```python
from build123d import *

# Parameters (mm, degrees)
CUT_EXTRUDE1_DEPTH = 2.413


with BuildPart() as part:
    # Sketch3 → Revolve1 (revolve)
    with BuildSketch(Plane(origin=(0, 0, 0), x_dir=(0, 0, -1), z_dir=(1, 0, 0))):
        Polygon((10.3505, 0), (-10.3505, 0), (-10.3505, 3.48615), (-9.8679, 3.96875), (-6.0071, 3.96875), (-5.5245, 3.48615), (-5.5245, 2.413), (9.609666667, 2.413), (10.3505, 1.672166667), align=None)
    revolve(axis=Axis((0, 0, -10.3505), (0, 0, 1)))

    # Sketch4 → Cut-Extrude1 (cut)
    with BuildSketch(Plane.XY.offset(10.3505)):
        Polygon((0, -2.291358881), (1.984375, -1.14567944), (1.984375, 1.14567944), (0, 2.291358881), (-1.984375, 1.14567944), (-1.984375, -1.14567944), align=None)
    extrude(amount=-CUT_EXTRUDE1_DEPTH, mode=Mode.SUBTRACT)

    # Cut-Extrude3 cone 1 section (through the dimple's axis) → Cut-Extrude3 (revolve, cut)
    with BuildSketch(Plane(origin=(0, 0, 10.3505), x_dir=(0, -1, 0), z_dir=(1, 0, 0))):
        Polygon((0, 0), (2.291358881, 0), (0, 2.291358881), align=None)
    revolve(axis=Axis((0, 0, 10.3505), (0, 0, -1)), mode=Mode.SUBTRACT)


solid = part.part
```
Could you check a few things on this model? Use its own coordinates, in mm. A direction names the side the tool comes from. Round coordinates to 2 decimals unless told otherwise and drop trailing zeros. Loops run counter-clockwise (first coordinate to the right, second up) from the corner with the lowest first, then second, coordinate; pieces in that order, holes last. Notation, with made-up numbers: M 11.5,-31.75 L 52.5,-31.75 A23 cw 52.5,5.25 Z; hole C 61,54.25 d1. An arc over 180 degrees is marked long. Answer as CSV lines item,"result".
1) For pin 1 Ø2 at (y, z) = (-3, -0.5) entering from +X, with a flat end and sliding along its axis, tell me the tip position at first contact or that it passes through.
From the geometry:
pin 1,"x = 1.35"
2) Imagine slicing it at A-A on y = 0. List the corners of the cut face in (x, z) for me.
From the geometry:
outline,"M -3.97,6.01 L -3.49,5.52 L -2.41,5.52 L -2.41,-9.61 L -1.67,-10.35 L 1.67,-10.35 L 2.41,-9.61 L 2.41,5.52 L 3.49,5.52 L 3.97,6.01 L 3.97,9.87 L 3.49,10.35 L 2.29,10.35 L 1.98,10.04 L 1.98,7.94 L -1.98,7.94 L -1.98,10.04 L -2.29,10.35 L -3.49,10.35 L -3.97,9.87 Z"
3) We'd pull the mould along X, two halves only. Please class faces 1 (the conical face through (-1.08, 1.84, 10.19)), 2 (the flat face through (0, 0, 7.938)), 3 (the flat face through (0, 0, -10.35)), 4 (the cylindrical face through (1.468, -1.915, -2.149)): released by +X, released by -X, zero draft, split by the parting line, or undercut.
From the geometry:
face 1,"undercut"
face 2,"undercut"
face 3,"zero draft"
face 4,"split by the parting line"
4) Which directions (+Z, -Z, +X, -X, +Y, -Y) give clear straight access to the entire face, cutting with the end or side of a thin tool? Please do faces 5 (the conical face through (1.08, -1.84, 10.19)), 6 (the cylindrical face through (3.874, -0.86, 7.91)).
From the geometry:
face 5,"+Z"
face 6,"+Z, -Z"
5) If I drill on probe 1 along Y at (x, z) = (0.75, -2.75); probe 2 along Y at (x, z) = (-0.25, 9); probe 3 along X at (y, z) = (0, -7.5), over which ranges is the centre line in solid material (lowest first)?
From the geometry:
probe 1,"-2.29 to 2.29"
probe 2,"-3.96 to -2.15, 2.15 to 3.96"
probe 3,"-2.41 to 2.41"
6) Imagine slicing it at B-B on z = 3.25. List the corners of the cut face in (x, y) for me.
From the geometry:
outline,"C 0,0 d4.83"
